```python
from build123d import *

# Parameters (mm, degrees)
F0_W     = 42
F0_H     = 42
F1_DEPTH = 40
F2_R     = 11
F3_DEPTH = 2
F4_R     = 2.5
F5_DEPTH = 21
F6_R     = 1.5
F7_DEPTH = 4.5
F8_SIZE  = 5


with BuildPart() as f1:
    # F0 (on Top) → F1 (new body)
    with BuildSketch(Plane.XY):
        Rectangle(F0_W, F0_H)
    extrude(amount=F1_DEPTH)

    # F2 (on face) → F3 (join)
    with BuildSketch(Plane.XY.offset(40)):
        Circle(F2_R)
    extrude(amount=F3_DEPTH)

    # F4 (on face) → F5 (join)
    with BuildSketch(Plane.XY.offset(42)):
        Circle(F4_R)
    extrude(amount=F5_DEPTH)

    # F6 (on face) → F7 (cut)
    with BuildSketch(Plane.XY.offset(40)):
        with Locations((-15.5, 15.5)):
            Circle(F6_R)
        with Locations((-15.5, -15.5)):
            Circle(F6_R)
        with Locations((15.5, 15.5)):
            Circle(F6_R)
        with Locations((15.5, -15.5)):
            Circle(F6_R)
    extrude(amount=-F7_DEPTH, mode=Mode.SUBTRACT)

    # F8
    f8_edges = [f1.edges().sort_by_distance(p)[0] for p in [
        (21, 21, 20),
        (21, -21, 20),
        (-21, -21, 20),
        (-21, 21, 20),
    ]]
    chamfer(f8_edges, length=F8_SIZE)


solid = f1.part
```
For this review, take the finished solid that the model builds, in its own axes (mm). A direction names the side the tool comes from. Round coordinates to 2 decimals unless told otherwise and drop trailing zeros. Write each loop counter-clockwise with the first axis right and the second up, starting at its lowest first coordinate (ties: lowest second). Pieces come first, ordered by that corner, then holes. Notation, with made-up numbers: (12, 8) -> (24, 8) arc R25 cw to (24, 41) -> close; hole circle Ø7 at (77.25, -7). An arc over 180 degrees is marked (long way). Use one line per item in the form item = value.
1) Take a section at D-D, the plane x = -9. Write out the cut boundary in (y, z).
Found:
outline = (-21, 0) -> (21, 0) -> (21, 40) -> (6.32, 40) -> (6.32, 42) -> (-6.32, 42) -> (-6.32, 40) -> (-21, 40) -> close
2) To check wall thickness, follow L1, parallel to Y at x = -15.5, z = 37.35; L2, parallel to X at y = -15, z = 38; L3, parallel to Z at x = 3, y = 13. State the ranges of each line that lie inside material, in increasing order. Write a range as from..to.
Found:
L1 = -21..-17, -14..14, 17..21
L2 = -21..-16.91, -14.09..14.09, 16.91..21
L3 = 0..40
3) Take a section at C-C, the plane z = 26.5. Write out the cut boundary in (x, y).
Found:
outline = (-21, -16) -> (-16, -21) -> (16, -21) -> (21, -16) -> (21, 16) -> (16, 21) -> (-16, 21) -> (-21, 16) -> close
4) Clearance check with flat-ended pins moving along their axes: pin 1 (1.5 mm diameter, centred on x = 16, y = -16, fed in from +Z); pin 2 (12 mm diameter, centred on x = 6.5, z = 56.5, fed in from +Y); pin 3 (4 mm diameter, centred on x = 15.5, y = -15.5, fed in from +Z). State where each tip first meets the part, or that it passes through.
Found:
pin_1 = 35.5
pin_2 = 2.45
pin_3 = 40
5) Take a section at A-A, the plane y = 0. Write out the cut boundary in (x, z).
Found:
outline = (-21, 0) -> (21, 0) -> (21, 40) -> (11, 40) -> (11, 42) -> (2.5, 42) -> (2.5, 63) -> (-2.5, 63) -> (-2.5, 42) -> (-11, 42) -> (-11, 40) -> (-21, 40) -> close
6) Tool access review of faces 5 (the flat face through (0, 21, 20)), 6 (the cylindrical face through (-2.38, -10.74, 40.99)): name each direction out of +Z, -Z, +X, -X, +Y, -Y from which nothing blocks a thin tool from reaching the whole face with its end or side.
Found:
face_5 = +Z, -Z, +X, -X, +Y
face_6 = +Z
7) Mouldability with a two-part tool opening along Y and no side actions: class faces 1 (the cylindrical face through (-17, 15.57, 37.78)), 2 (the flat face through (19, -18, 20)), 3 (the flat face through (-16, 16, 35.5)), 4 (the flat face through (-3, 0, 42)) as +Y half, -Y half, draft (parallel to the pull), parting line (faces both ways), or undercut.
Found:
face_1 = undercut
face_2 = -Y half
face_3 = undercut
face_4 = draft
